Read the model definition and answer for the solid it produces. Units are mm, in the model's axes. A direction names the side the tool comes from. Coordinates: 2 decimals unless noted, no trailing zeros. Loops run counter-clockwise (first coordinate to the right, second up) from the corner with the lowest first, then second, coordinate; pieces in that order, holes last. Notation, with made-up numbers: M 72,-3.75 L 130,-3.75 A17 cw 130,21.25 Z; hole C -16,-14 d4. An arc over 180 degrees is marked long. One line per item, written item: value. Start each with the question number.
```python
from build123d import *

# Parameters (mm, degrees)
F1_DEPTH  = 25.4
F3_DEPTH  = 2.778125
F5_D      = 3.556
F7_DEPTH  = 1.5875
F9_R      = 10.16
F10_R     = 10.16
F11_R     = 2.54
F12_R     = 5.08
F13_D     = 2.8448
F13_DEPTH = 19.05
F13_TIP   = 0.8546641445


with BuildPart() as f1:
    # F0 (on Front) → F1 (new body)
    with BuildSketch(Plane.XZ):
        with BuildLine():
            Line((-3.269999937, 50.5886303798), (-3.269999937, 25.1886303798))
            Line((-3.269999937, 25.1886303798), (-12.8627581622, 21.9022704864))
            Line((-12.8627581622, 21.9022704864), (-60.48375, 5.5879098004))
            Line((-60.48375, 5.5879098004), (-60.48375, 18.2879098004))
            Line((-60.48375, 18.2879098004), (-62.865, 18.2879098004))
            Line((-62.865, 18.2879098004), (-62.865, 6.3181702256))
            Line((-62.865, 6.3181702256), (-62.865, 4.7199768273))
            ThreePointArc((-62.865, 4.7199768273), (-63.5, -4.7625), (-64.135, 4.7199768273))
            Line((-64.135, 4.7199768273), (-64.135, 6.3181702256))
            Line((-64.135, 6.3181702256), (-64.135, 18.2879098004))
            Line((-64.135, 18.2879098004), (-66.51625, 18.2879098004))
            Line((-66.51625, 18.2879098004), (-66.51625, 5.5879098004))
            ThreePointArc((-66.51625, 5.5879098004), (-69.0879098004, -3.01625), (-60.48375, -5.5879098004))
            Line((-60.48375, -5.5879098004), (-8.4538247205, -23.9518860968))
            ThreePointArc((-8.4538247205, -23.9518860968), (24.7065902088, -5.894438078), (3.269999937, 25.1886303798))
            Line((3.269999937, 25.1886303798), (3.269999937, 50.5886303798))
            Line((3.269999937, 50.5886303798), (1.27, 50.5886303798))
            Line((1.27, 50.5886303798), (1.27, 25.3682301314))
            Line((1.27, 25.3682301314), (1.27, 20.2802736668))
            ThreePointArc((1.27, 20.2802736668), (0, -20.32), (-1.27, 20.2802736668))
            Line((-1.27, 20.2802736668), (-1.27, 25.3682301314))
            Line((-1.27, 25.3682301314), (-1.27, 50.5886303798))
            Line((-1.27, 50.5886303798), (-3.269999937, 50.5886303798))
        make_face()
    extrude(amount=F1_DEPTH)

    # F2 (on face) → F3 (cut)
    with BuildSketch(Plane.YZ.offset(3.269999937)):
        Polygon((-10.353648506, 33.8246303798), (-8.007297012, 37.8886303798), (-10.353648506, 41.9526303798), (-15.046351494, 41.9526303798), (-17.392702988, 37.8886303798), (-15.046351494, 33.8246303798), align=None)
    extrude(amount=-F3_DEPTH, mode=Mode.SUBTRACT)

    # F5 (through all)
    with Locations(Plane.YZ.offset(3.269999937)):
        with Locations((-12.693702988, 37.8886303798)):
            Hole(F5_D / 2)

    # F6 (on face) → F7 (cut)
    with BuildSketch(Plane(origin=(-66.51625, 0, 0), x_dir=(0, -1, 0), z_dir=(-1, 0, 0))):
        Polygon((10.8669128953, 8.7629098004), (14.5330871047, 8.7629098004), (16.3661742094, 11.9379098004), (14.5330871047, 15.1129098004), (10.8669128953, 15.1129098004), (9.0338257906, 11.9379098004), align=None)
    extrude(amount=-F7_DEPTH, mode=Mode.SUBTRACT)

    # F9
    f9_edges = [f1.edges().sort_by_distance(p)[0] for p in [
        (-3.27, -12.7, 25.18863),
    ]]
    fillet(f9_edges, radius=F9_R)

    # F10
    f10_edges = [f1.edges().sort_by_distance(p)[0] for p in [
        (3.27, -12.7, 25.18863),
    ]]
    fillet(f10_edges, radius=F10_R)

    # F11
    f11_edges = [f1.edges().sort_by_distance(p)[0] for p in [
        (-60.48375, -12.7, 5.58791),
    ]]
    fillet(f11_edges, radius=F11_R)

    # F12
    f12_edges = [f1.edges().sort_by_distance(p)[0] for p in [
        (-66.51625, -12.7, 5.58791),
    ]]
    fillet(f12_edges, radius=F12_R)

    # F13
    with Locations(Plane(origin=(-64.92875, 0, 0), x_dir=(0, -1, 0), z_dir=(-1, 0, 0))):
        with Locations((12.6853353032, 11.9633098004)):
            Hole(F13_D / 2, depth=F13_DEPTH)
            with Locations((0, 0, -(F13_DEPTH + F13_TIP / 2))):  # 118° drill point
                Cone(0, F13_D / 2, F13_TIP, mode=Mode.SUBTRACT)


solid = f1.part
```
1) Section A-A (z = 0) is taken. Determine the outline of the cut face in (x, y), then the cut area to 3 significant figures.
2) Section C-C (x = 0) is taken. Determine the outline of the cut face in (y, z).
3) A tool of negligible diameter and unlimited length cuts with its end or side. For faces 1 (the face through (-64.135, -13, 10)), 2 (the face through (3.27, -13, 44)), 3 (the face through (-65, -13, 18.288)), 4 (the face through (-61.658, -13.814, 11.098)), from which of +Z, -Z, +X, -X, +Y, -Y can it reach the whole face along a straight path? Write none if from no direction.
4) For a pull along X with two mould halves and no side action, classify faces 5 (the face through (-60.484, -13, 14)), 6 (the face through (-2, -13, 50.589)), 7 (the face through (-66.891, -12.878, 6.154)) as released by +X, released by -X, zero draft, split by the parting line, or undercut.
5) Section D-D (x = -50) is taken. Determine the outline of the cut face in (y, z).
6) Consider line 1 along X through (y, z) = (-5, 35.5); line 2 along X through (y, z) = (-15.75, 3); line 3 along X through (y, z) = (-12, 0). Determine where each line is inside the solid, lowest interval first.
7) Flat-ended cylindrical pins translate along their axes: pin 1 (2 mm diameter, centred on y = -15, z = 28.5, fed in from +X); pin 2 (1.3 mm diameter, centred on x = -66, y = -13.5, fed in from +Z); pin 3 (15 mm diameter, centred on x = -63.5, z = 0, fed in from -Y); pin 4 (4.5 mm diameter, centred on y = -12.5, z = 14.5, fed in from +X). Find the tip coordinate at first contact, or state that the pin passes through.
Results found:
1. outline: M -69.85,-25.4 L -68.26,-25.4 L -68.26,0 L -69.85,0 Z; M -58.74,-25.4 L -20.32,-25.4 L -20.32,0 L -58.74,0 Z; M 20.32,-25.4 L 25.4,-25.4 L 25.4,0 L 20.32,0 Z
1. area: 1,150 mm²
2. outline: M -25.4,-25.4 L 0,-25.4 L 0,-20.32 L -25.4,-20.32 Z
3. face 1: +Z, +Y, -Y
3. face 2: +Z, +X, +Y, -Y
3. face 3: +Z, -X, +Y, -Y
3. face 4: -X
4. face 5: undercut
4. face 6: zero draft
4. face 7: released by -X
5. outline: M -25.4,-9.29 L 0,-9.29 L 0,9.18 L -25.4,9.18 Z
6. line 1: x = -3.27 to -1.27, 1.27 to 3.27
6. line 2: x = -69.1 to -67.2, -59.8 to -20.1, 20.1 to 25.22
6. line 3: x = -69.85 to -68.26, -58.74 to -20.32, 20.32 to 25.4
7. pin 1: stops at x = 4.84
7. pin 2: stops at z = 18.29
7. pin 3: stops at y = -25.4
7. pin 4: stops at x = 22.25
